Input: part model. Units: mm. Frame: model coordinates. A direction names the side the tool comes from. Round coordinates to 2 decimals unless told otherwise and drop trailing zeros. Loops run counter-clockwise (first coordinate to the right, second up) from the corner with the lowest first, then second, coordinate; pieces in that order, holes last.
(1) Line query: line 1 (X direction, y = 7.25, z = 70); line 2 (Y direction, x = -47, z = 122); line 3 (X direction, y = -1, z = 70). Output: solid intervals per line, ascending.
(2) Cut plane B-B, the plane z = 84. Output: boundary loops of the cut face in (x, y).
(3) Cut plane D-D, the plane y = 13. Output: boundary loops of the cut face in (x, z).
(4) First-contact query: pin 1 Ø10 at (y, z) = (120, 14.5) entering from +X; pin 2 Ø9 at (x, y) = (-76, -0.5) entering from -Z; pin 3 Ø3 at (y, z) = (66, 122.5) entering from +X. Flat tips, straight axial feed; report the tip coordinate or a pass-through.
(5) Access query for faces 1 (the face through (-132, 72.7, 123)), 2 (the face through (-64, 0, 69)), 3 (the face through (-67.055, 5.07, 68.301)). Directions: +Z, -Z, +X, -X, +Y, -Y. A direction counts if a zero-diameter tool reaches every point of the face in a straight line with its end or side. Return the directions, or none.
(6) Cut plane A-A, the plane x = 10. Output: boundary loops of the cut face in (y, z).
(7) Cut plane C-C, the plane z = 41. Output: boundary loops of the cut face in (x, y).
(8) Draft query along Y for faces 4 (the face through (-118, 56, 123)), 5 (the face through (8.856, -0.424, 43.366)), 6 (the face through (-72, 10, 61)). Return one class per face: released by +Y, released by -Y, zero draft, split by the parting line, or undercut.
Autodesk Inventor part; units mm, degrees
ref_plane "YZ Plane" through (0, 0, 0) normal (1, 0, 0) x (0, 1, 0)
ref_plane "XZ Plane" through (0, 0, 0) normal (0, 1, 0) x (-1, 0, 0)
ref_plane "XY Plane" through (0, 0, 0) normal (0, 0, 1) x (1, 0, 0)
sketch "Sketch1" plane through (0, 0, 0) normal (0, 1, 0) x (-1, 0, 0)
  line L0 (0, 0) -> (150, 0)
  line L1 (150, 0) -> (150, 125)
  line L2 (150, 125) -> (0, 125)
  line L3 (0, 125) -> (0, 0)
  dimension "d0" = 150
  dimension "d1" = 125
extrude "Extrusion1" add sketch "Sketch1" along normal blind 10
sketch "Sketch2" plane through (0, 10, 0) normal (0, 1, 0) x (1, 0, 0)
  line L0 (0, -125) -> (0, 0)
  line L1 (0, 0) -> (-146, 0)
  line L2 (-146, 0) -> (-146, -121)
  line L3 (-146, -121) -> (0, -121)
  line L4 (0, -121) -> (0, 0)
  line L5 (0, -125) -> (0, 0)
  line L6 (0, 0) -> (-150, 0)
  line L7 (-150, 0) -> (-150, -125)
  line L8 (-150, -125) -> (0, -125)
  point P0 (-146, 0)
  dimension "d4" = 146
  dimension "d5" = 121
extrude "Extrusion2" add sketch "Sketch2" along normal blind 125 contours L8 L7 L6 L2 L3 L0
sketch "Sketch3" plane through (0, 0, 125) normal (1, 0, 0) x (0, 0, -1)
  line L0 (0, 0) -> (0, 135)
  line L1 (0, 0) -> (0, 5)
  line L2 (125, 0) -> (125, 10)
  line L3 (125, 0) -> (0, 0)
  line L4 (125, 0) -> (0, 0)
  line L5 (0, 5) -> (115, 5)
  line L6 (115, 5) -> (125, 5)
  line L7 (115, 5) -> (115, 0)
  line L8 (0, 0) -> (125, 0)
  dimension "d8" = 5
  dimension "d95" = 125
  dimension "d96" = 115
sketch "Sketch4" plane through (0, 10, 121) normal (0, 0, -1) x (-1, 0, 0)
  line L0 (0, 20) -> (16, 20)
  line L1 (16, 20) -> (32.7, 20)
  line L2 (32.7, 20) -> (32.7, 32.9)
  line L3 (32.7, 32.9) -> (16, 32.9)
  line L4 (16, 32.9) -> (16, 20)
  line L5 (16, 26.45) -> (13, 26.45)
  line L6 (13, 26.45) -> (11.5, 26.45)
  circle A0 centre (11.5, 26.45) radius 1.5
  line L7 (32.7, 26.45) -> (37.2, 26.45)
  circle A1 centre (37.2, 26.45) radius 1.5
  line L8 (16, 32.9) -> (16, 47.9)
  line L9 (16, 47.9) -> (32.7, 47.9)
  line L10 (32.7, 47.9) -> (32.7, 60.8)
  line L11 (32.7, 60.8) -> (16, 60.8)
  line L12 (16, 60.8) -> (16, 47.9)
  line L13 (16, 54.35) -> (11.5, 54.35)
  line L14 (11.5, 54.35) -> (37.2, 54.35)
  circle A2 centre (11.5, 54.35) radius 1.5
  circle A3 centre (37.2, 54.35) radius 1.5
  line L15 (47.2, 54.35) -> (51.7, 54.35)
  line L16 (51.7, 54.35) -> (51.7, 47.9)
  line L17 (51.7, 47.9) -> (68.4, 47.9)
  line L18 (68.4, 47.9) -> (68.4, 60.8)
  line L19 (68.4, 60.8) -> (51.7, 60.8)
  line L20 (51.7, 60.8) -> (51.7, 54.35)
  line L21 (68.4, 54.35) -> (72.9, 54.35)
  circle A4 centre (47.2, 54.35) radius 1.5
  circle A5 centre (72.9, 54.35) radius 1.5
  line L22 (0, 0) -> (0, 125)
  line L23 (0, 20) -> (0, 0)
  line L24 (51.7, 32.9) -> (51.7, 20)
  line L25 (51.7, 20) -> (68.4, 20)
  line L26 (68.4, 20) -> (68.4, 32.9)
  line L27 (68.4, 32.9) -> (51.7, 32.9)
  line L28 (68.4, 26.45) -> (72.9, 26.45)
  line L29 (72.9, 26.45) -> (47.2, 26.45)
  circle A6 centre (47.2, 26.45) radius 1.5
  circle A7 centre (72.9, 26.45) radius 1.5
  line L30 (68.4, 47.9) -> (68.4, 32.9)
  line L31 (37.2, 54.35) -> (47.2, 54.35)
  point P0 (0, -10)
  dimension "d12" = 16
  dimension "d13" = 16.7
  dimension "d14" = 12.9
  dimension "d15" = 3
  dimension "d16" = 1.5
  dimension "d17" = 4.5
  dimension "d18" = 3
  dimension "d19" = 15
  dimension "d20" = 12.9
  dimension "d23" = 4.5
  dimension "d25" = 4.5
  dimension "d29" = 3
  dimension "d30" = 3
  dimension "d57" = 20
  dimension "d58" = 3
  dimension "d59" = 3
  dimension "d60" = 16.7
  dimension "d62" = 15
  dimension "d73" = 3
  dimension "d74" = 10
  dimension "d75" = 4.5
  dimension "d76" = 16.7
  dimension "d77" = 16.7
extrude "Extrusion4" cut sketch "Sketch4" against normal blind 125 contours L4 L3 L2 L1 | L26 L29 L24 L27 | L20 L19 L18 L17 L16 | L12 L14 L10 L9 | L12 L11 L10 L14 | L26 L25 L24 L29
hole "Hole1" at (-11.5, 64.35, 121) at (-37.2, 64.35, 121) at (-47.2, 64.35, 121) at (-72.9, 64.35, 121) at (-37.2, 36.45, 121) at (-11.5, 36.45, 121) at (-47.2, 36.45, 121) at (-72.9, 36.45, 121) direction (0, 0, 1) diameter 3 end through all
sketch "Sketch5" plane through (-150, 135, 125) normal (0, 0, 1) x (1, 0, 0)
  circle A0 centre (77.1, -70.65) radius 1.5
  line L0 (77.1, -70.65) -> (65.6, -70.65)
  line L1 (65.6, -70.65) -> (65.6, -62.3)
  line L2 (65.6, -62.3) -> (65.6, -79)
  line L3 (65.6, -79) -> (57.5, -79)
  line L4 (57.5, -79) -> (57.5, -62.3)
  line L5 (57.5, -62.3) -> (65.6, -62.3)
  line L6 (57.5, -62.3) -> (51.1, -62.3)
  line L7 (51.1, -62.3) -> (36.6, -62.3)
  line L8 (51.1, -62.3) -> (43, -62.3)
  line L9 (43, -62.3) -> (43, -79)
  line L10 (43, -79) -> (51.1, -79)
  line L11 (51.1, -79) -> (51.1, -62.3)
  line L12 (36.6, -62.3) -> (28.5, -62.3)
  line L13 (28.5, -62.3) -> (28.5, -79)
  line L14 (28.5, -79) -> (36.6, -79)
  line L15 (36.6, -79) -> (36.6, -62.3)
  line L16 (28.5, -62.3) -> (22.1, -62.3)
  line L17 (22.1, -62.3) -> (14, -62.3)
  line L18 (14, -62.3) -> (14, -79)
  line L19 (14, -79) -> (22.1, -79)
  line L20 (22.1, -79) -> (22.1, -62.3)
  point P0 (150, -135)
  point P1 (43, -62.3)
  dimension "d41" = 11.5
  dimension "d43" = 8.35
  dimension "d44" = 16.7
  dimension "d45" = 8.1
  dimension "d46" = 6.4
  dimension "d47" = 14.5
  dimension "d48" = 8.1
  dimension "d49" = 16.7
  dimension "d50" = 8.1
  dimension "d51" = 16.7
  dimension "d52" = 6.4
  dimension "d53" = 8.1
  dimension "d54" = 16.7
extrude "Extrusion5" cut sketch "Sketch5" against normal blind 10 contours L20 L19 L18 L17 | L15 L14 L13 L12 | L11 L10 L9 L7 | L2 L3 L4 L5 L1
sketch "Sketch8" plane through (-150, 135, 125) normal (0, 0, 1) x (1, 0, 0)
  circle A0 centre (77.1, -98.55) radius 1.5
  line L0 (77.1, -98.55) -> (65.6, -98.55)
  line L1 (65.6, -98.55) -> (65.6, -87.25)
  line L2 (65.6, -87.25) -> (65.6, -109.85)
  line L3 (65.6, -109.85) -> (53.1, -109.85)
  line L4 (53.1, -109.85) -> (53.1, -87.25)
  line L5 (53.1, -87.25) -> (65.6, -87.25)
  line L6 (53.1, -87.25) -> (43.1, -87.25)
  line L7 (43.1, -87.25) -> (43.1, -109.85)
  line L8 (43.1, -109.85) -> (30.6, -109.85)
  line L9 (30.6, -109.85) -> (30.6, -87.25)
  line L10 (30.6, -87.25) -> (43.1, -87.25)
  line L11 (30.6, -87.25) -> (20.6, -87.25)
  line L12 (20.6, -87.25) -> (20.6, -109.85)
  line L13 (20.6, -109.85) -> (8.1, -109.85)
  line L14 (8.1, -109.85) -> (8.1, -87.25)
  line L15 (8.1, -87.25) -> (20.6, -87.25)
  dimension "d63" = 11.5
  dimension "d64" = 11.3
  dimension "d65" = 22.6
  dimension "d66" = 12.5
  dimension "d67" = 10
  dimension "d68" = 12.5
  dimension "d69" = 10
  dimension "d70" = 22.6
  dimension "d71" = 12.5
  dimension "d113" = 22.6
extrude "Extrusion6" cut sketch "Sketch8" against normal blind 10 contours L12 L13 L14 L15 | L7 L8 L9 L10 | L2 L3 L4 L5 L1
sketch "Sketch9" plane through (-146, 10, 121) normal (1, 0, 0) x (0, 0, -1)
  line L0 (0, 0) -> (0, 125)
  line L1 (0, 125) -> (50, 125)
  line L2 (0, 125) -> (121, 125)
  line L3 (50, 125) -> (50, 85)
  line L4 (50, 85) -> (95, 85)
  line L5 (95, 85) -> (95, 28)
  line L6 (95, 28) -> (50, 28)
  line L7 (50, 28) -> (50, 85)
  line L8 (72.5, 85) -> (72.5, 80)
  line L9 (72.5, 80) -> (72.5, 33)
  circle A0 centre (72.5, 80) radius 2.5
  circle A1 centre (72.5, 33) radius 2.5
  point P0 (121, -10)
  dimension "d80" = 50
  dimension "d81" = 40
  dimension "d82" = 45
  dimension "d83" = 57
  dimension "d84" = 5
  dimension "d85" = 47
  dimension "d86" = 5
  dimension "d87" = 5
hole "Hole2" at (-146, 90, 48.5) at (-146, 43, 48.5) direction (-1, 0, 0) diameter 4.318 end through all
extrude "Extrusion7" add sketch "Sketch3" along normal blind 20 contours L0 L5 L7 L3
sketch "Sketch10" plane through (0, 0, 0) normal (0, -1, 0) x (1, 0, 0)
  point P0 (0, 0)
sketch "Sketch11" plane through (0, 0, 0) normal (0, 0, -1) x (-1, 0, 0)
  line L0 (150, 0) -> (150, 135)
  line L1 (150, 0) -> (150, 5)
  line L2 (150, 5) -> (10, 5)
  line L3 (10, 5) -> (10, 0)
  line L4 (10, 0) -> (150, 0)
  point P0 (0, 0)
  dimension "d99" = 5
  dimension "d100" = 140
extrude "Extrusion8" cut sketch "Sketch11" against normal blind 20
sketch "Sketch13" plane through (0, 10, 0) normal (0, 1, 0) x (1, 0, 0)
  line L0 (0, 0) -> (-146, 0)
  line L1 (0, 0) -> (-10, 0)
  line L2 (-10, 0) -> (-55.3333, 0)
  line L3 (-55.3333, 0) -> (-100.6667, 0)
  line L4 (-100.6667, 0) -> (-100.6667, -10)
  line L5 (-55.3333, 0) -> (-55.3333, -10)
  dimension "d114" = 10
  dimension "d115" = 45.3333
  dimension "d116" = 45.3333
  dimension "d117" = 10
  dimension "d118" = 10
hole "Hole4" at (-100.6667, 10, 10) at (-55.3333, 10, 10) direction (0, -1, 0) diameter 4.318 end through all
sketch "Sketch12" plane through (0, 0, 0) normal (0, 1, 0) x (1, 0, 0)
  line L0 (-146, -121) -> (-146, 0)
  line L1 (-146, 0) -> (-106, 0)
  line L2 (0, 0) -> (-146, 0)
  line L3 (-106, 0) -> (-106, -70)
  line L4 (-106, -70) -> (-66, -70)
  dimension "d103" = 40
  dimension "d104" = 70
  dimension "d105" = 40
hole "Hole3" at (-66, 0, 70) at (-106, 0, 70) direction (0, 1, 0) diameter 4 end through all counterbore diameter 6 counterbore depth 3
sketch "Sketch16" plane through (0, 0, 0) normal (0, -1, 0) x (1, 0, 0)
  circle A0 centre (-66, 70) radius 3
  circle A1 centre (-106, 70) radius 3
  line L0 (-10, 20) -> (-10, 0)
  line L1 (0, 0) -> (-10, 0)
  line L2 (0, 10) -> (0, 0)
  line L3 (0, 10) -> (20, 10)
  line L4 (20, 125) -> (20, 10)
  line L5 (-150, 125) -> (20, 125)
  line L6 (-150, 20) -> (-150, 125)
  line L7 (-150, 20) -> (-10, 20)
extrude "Extrusion10" add sketch "Sketch16" along normal blind 3
sketch "Sketch17" plane through (-66, 3, 70) normal (0, -1, 0) x (1, 0, 0)
  circle A0 centre (0, 0) radius 3
  circle A1 centre (0, 0) radius 2
  circle A2 centre (-40, 0) radius 3
  circle A3 centre (-40, 0) radius 2
  point P0 (66, -70)
extrude "Extrusion11" add sketch "Sketch17" along normal blind 3
sketch "Sketch18" plane through (0, -3, 0) normal (0, -1, 0) x (1, 0, 0)
  circle A0 centre (10, 84) radius 1.75
  circle A1 centre (10, 84) radius 1.75
  circle A2 centre (10, 47) radius 1.75
  circle A3 centre (10, 47) radius 1.75
  point P0 (0, 0)
hole "Hole6" at (10, -3, 47) at (10, -3, 84) direction (0, 1, 0) diameter 4.318 end through all counterbore diameter 7.62 counterbore depth 5.08
properties part number "Quarter4"
Reported:
1. line 1: x = -150 to -108, -104 to -68, -64 to 0
1. line 2: y = -3 to 34.96, 37.94 to 62.86, 65.84 to 135
1. line 3: x = -150 to -109, -103 to -69, -63 to 20
2. outline: (-150, -3) - (6.19, -3) - (6.19, 2.08) - (7.84, 2.08) - (7.84, 5) - (0, 5) - (0, 10) - (-146, 10) - (-146, 135) - (-150, 135) - close; (12.16, 2.08) - (13.81, 2.08) - (13.81, -3) - (20, -3) - (20, 5) - (12.16, 5) - close
3. outline: (-150, 0) - (-146, 0) - (-146, 121) - (0, 121) - (0, 125) - (-150, 125) - close
4. pin 1: stops at x = -146
4. pin 2: stops at z = 20
4. pin 3: stops at x = 0
5. face 1: +Z, -Z
5. face 2: -Y
5. face 3: +Y, -Y
6. outline: (-3, 10) - (5, 10) - (5, 44.84) - (2.08, 44.84) - (2.08, 43.19) - (-3, 43.19) - close; (-3, 50.81) - (2.08, 50.81) - (2.08, 49.16) - (5, 49.16) - (5, 81.84) - (2.08, 81.84) - (2.08, 80.19) - (-3, 80.19) - close; (-3, 87.81) - (2.08, 87.81) - (2.08, 86.16) - (5, 86.16) - (5, 125) - (-3, 125) - close
7. outline: (-150, -3) - (20, -3) - (20, 5) - (0, 5) - (0, 10) - (-146, 10) - (-146, 135) - (-150, 135) - close
8. face 4: undercut
8. face 5: zero draft
8. face 6: released by +Y
